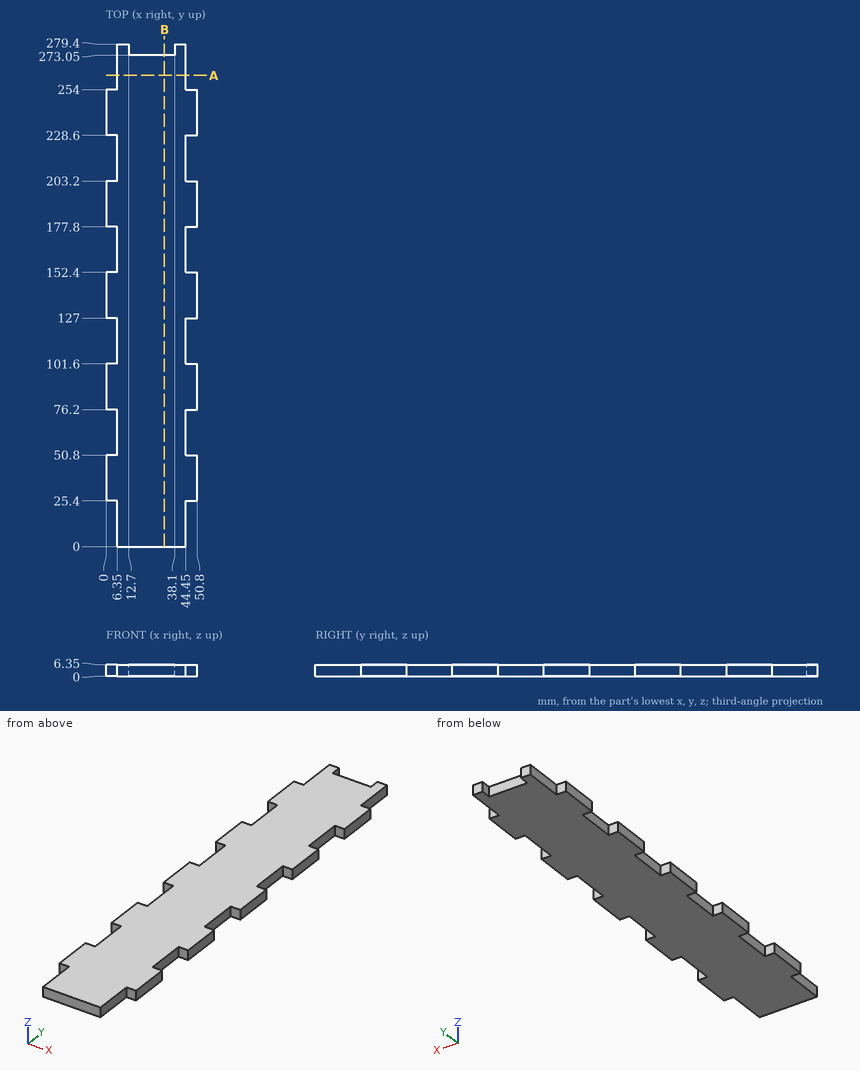
Part print with two shaded views. Sizes in mm from the minimum x, y, z corner. Coordinates: 2 decimals unless noted, no trailing zeros. Write each loop counter-clockwise with the first axis right and the second up, starting at its lowest first coordinate (ties: lowest second). Pieces come first, ordered by that corner, then holes. Notation, with made-up numbers: (62.25, 2) - (71.25, 2) arc R30 cw to (71.25, 26) - close; hole circle Ø7 at (-25.5, 59). An arc over 180 degrees is marked (long way). Put each result on its own line as item: value.
1. Band-saw the part on A-A (y = 262). Write the cut outline in (x, z), then the cut area to 3 significant figures.
Final values:
outline: (6.35, 0) - (44.45, 0) - (44.45, 6.35) - (6.35, 6.35) - close
area: 242 mm²
2. Band-saw the part on B-B (x = 32.5). Write the cut outline in (y, z).
Final values:
outline: (0, 0) - (273.05, 0) - (273.05, 6.35) - (0, 6.35) - close
3. Probe line 1 along Y through (x, z) = (46, 1.5); line 2 along X through (y, z) = (60, 1); line 3 along Y through (x, z) = (30, 4.25). List the from-to ranges inside material, lowest first. Write a range as [from, to].
Final values:
line 1: y = [25.4, 50.8], [76.2, 101.6], [127, 152.4], [177.8, 203.2], [228.6, 254]
line 2: x = [6.35, 44.45]
line 3: y = [0, 273.05]
4. Flat gauge pins, fed straight in: pin 1 Ø3 at (x, z) = (47.5, 3) entering from -Y; pin 2 Ø1.5 at (x, y) = (33, 248.5) entering from -Z; pin 3 Ø1.5 at (x, y) = (45.5, 161.5) entering from -Z; pin 4 Ø1.9 at (y, z) = (68, 3.5) entering from +X. Where does each tip first touch, or does it go through?
Final values:
pin 1: stops at y = 25.4
pin 2: stops at z = 0
pin 3: passes through
pin 4: stops at x = 44.45
